Part print with two shaded views. Sizes in mm from the minimum x, y, z corner. Coordinates: 2 decimals unless noted, no trailing zeros. Write each loop counter-clockwise with the first axis right and the second up, starting at its lowest first coordinate (ties: lowest second). Pieces come first, ordered by that corner, then holes.
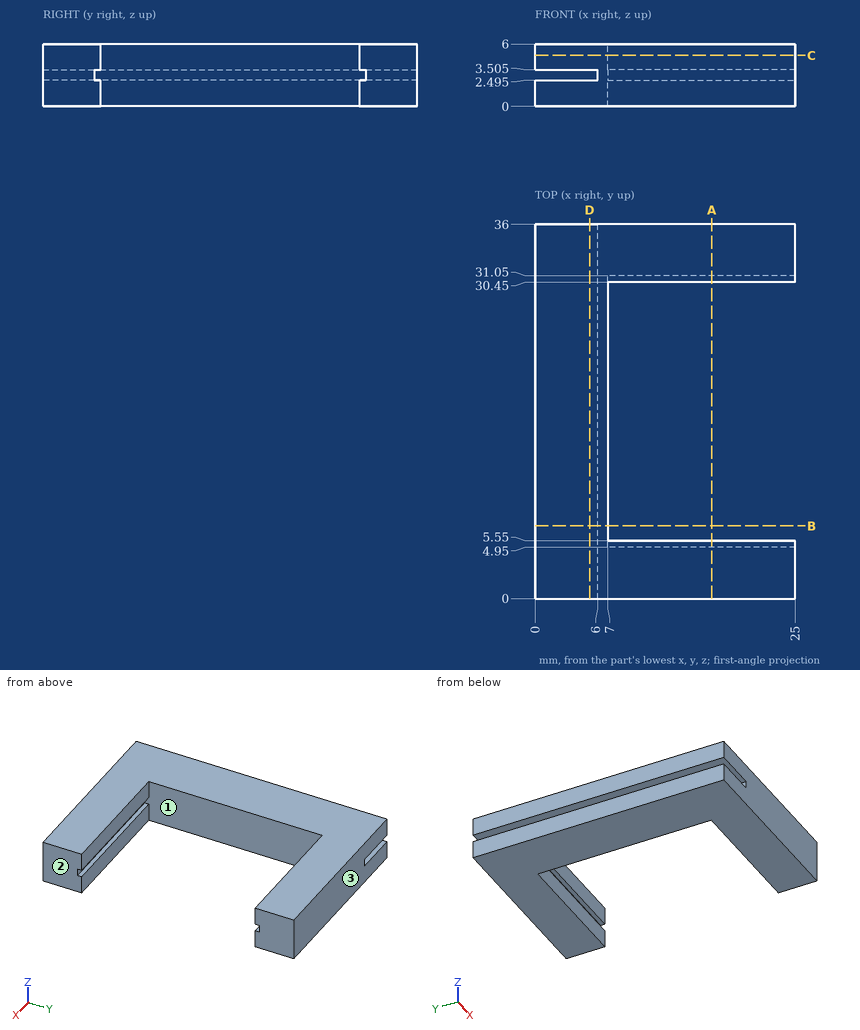
(1) Slice it at A-A, the plane x = 17. List the corners of the cut face in (y, z) (3 decimals).
(2) Two-plate mould, pull along Y, no slides. Class the marked faces 1, 2 and 3: pulls with the +Y half, pulls with the -Y half, needs draft (parallel to the pull), parting line crosses it, or undercut.
(3) Slice it at C-C, the plane z = 4.9. List the corners of the cut face in (x, y), and give its area (3 significant figures).
(4) Flat gauge pins, fed straight in: P1, Ø1, axis at y = 16.5, z = 3.5, coming from the +X side; P2, Ø0.8, axis at y = 16, z = 3, coming from the -X side. Where does each tip first touch, or does it go through?
(5) Slice it at D-D, the plane x = 5.25. List the corners of the cut face in (y, z) (3 decimals), and give its area (3 significant figures).
(6) Slice it at B-B, the plane y = 7. List the corners of the cut face in (x, z) (3 decimals), and give its area (3 significant figures).
(7) Probe L1, parallel to Y at x = 8.5, z = 3.85; L2, parallel to Z at x = 1, y = 21 (3 decimals); L3, parallel to X at y = 14, z = 1.6. List the from-to ranges inside material, lowest first.
Results:
1. outline: (0, 0) - (5.55, 0) - (5.55, 2.495) - (4.95, 2.495) - (4.95, 3.505) - (5.55, 3.505) - (5.55, 6) - (0, 6) - close; (30.45, 0) - (36, 0) - (36, 6) - (30.45, 6) - (30.45, 3.505) - (31.05, 3.505) - (31.05, 2.495) - (30.45, 2.495) - close
2. face 1: undercut
2. face 2: needs draft
2. face 3: pulls with the +Y half
3. outline: (0, 0) - (25, 0) - (25, 5.55) - (7, 5.55) - (7, 30.45) - (25, 30.45) - (25, 36) - (0, 36) - close
3. area: 452 mm2
4. P1: stops at x = 7
4. P2: stops at x = 6
5. outline: (0, 0) - (36, 0) - (36, 2.495) - (0, 2.495) - close; (0, 3.505) - (36, 3.505) - (36, 6) - (0, 6) - close
5. area: 180 mm2
6. outline: (0, 0) - (7, 0) - (7, 6) - (0, 6) - (0, 3.505) - (6, 3.505) - (6, 2.495) - (0, 2.495) - close
6. area: 35.9 mm2
7. L1: y = 0 to 5.55, 30.45 to 36
7. L2: z = 0 to 2.495, 3.505 to 6
7. L3: x = 0 to 7
